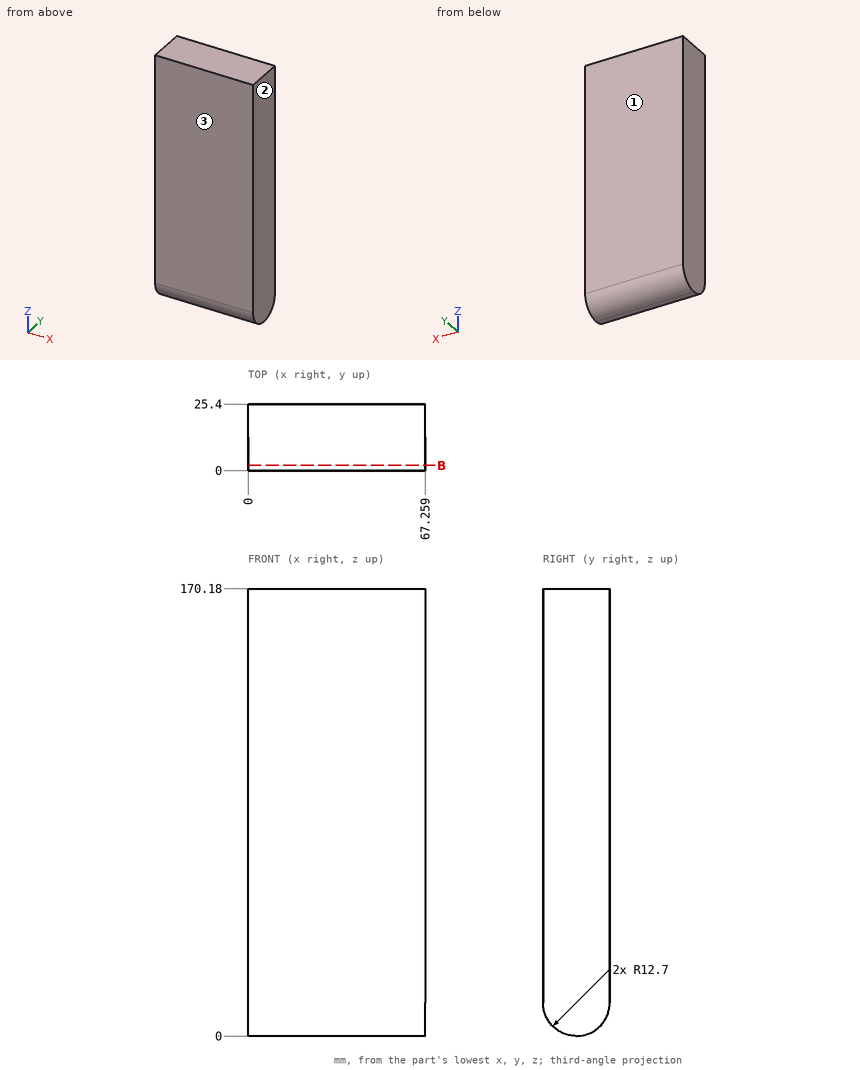
Answer from the drawing. Dimensions are ordinates in mm from the lowest x, y and z of the part. Round coordinates to 2 decimals unless told otherwise and drop trailing zeros. Loops run counter-clockwise (first coordinate to the right, second up) from the corner with the lowest first, then second, coordinate; pieces in that order, holes last.
(1) Find the intervals of material crossed by L1, parallel to Z at x = 20, y = 23; L2, parallel to Z at x = 49, y = 18.75 (1 decimal), in increasing order.
Computed values:
L1: z = 5.27 to 170.18
L2: z = 1.5 to 170.2
(2) The part is cut by section B-B, the plane y = 2. Give the vertices of the cut face in (x, z), and give its area (3 significant figures).
Computed values:
outline: (0, 5.86) - (67.26, 5.86) - (67.26, 170.18) - (0, 170.18) - close
area: 11,100 mm2
(3) Each of these flat-tipped pins is pushed along its axis until it touches: P1, Ø2, axis at x = 19.5, y = 17.5, coming from the -Z side; P2, Ø5, axis at x = 15, y = 17, coming from the -Z side; P3, Ø10, axis at x = 14, y = 5.5, coming from the -Z side. Where does it stop, or does it pass through?
Computed values:
P1: stops at z = 0.58
P2: stops at z = 0.13
P3: stops at z = 0.19
(4) The mould has two halves that part along Y. Classify the marked faces 1, 2 and 3: pulls with the +Y half, pulls with the -Y half, needs draft (parallel to the pull), parting line crosses it, or undercut.
Computed values:
face 1: pulls with the +Y half
face 2: needs draft
face 3: pulls with the -Y half
